```python
from build123d import *

# Parameters (mm, degrees)
EXTRUDE_1_DEPTH     = 5
EXTRUDE_2_DEPTH     = 15
CUT_EXTRUDE_1_DEPTH = 15


with BuildPart() as part:
    # 草圖1 → 填料-伸長1 (new body)
    with BuildSketch(Plane(origin=(0, 0, 0), x_dir=(1, 0, 0), z_dir=(0, 1, 0))):
        with BuildLine():
            ThreePointArc((-10, 5), (-15, 0), (-10, -5))
            Line((-10, -5), (0, -5))
            Line((0, -5), (0, -10))
            ThreePointArc((0, -10), (10, 0), (0, 10))
            Line((0, 10), (-5, 10))
            Line((-5, 10), (-5, 5))
            Line((-5, 5), (-10, 5))
        make_face()
    extrude(amount=EXTRUDE_1_DEPTH)

    # 草圖1<3> → 填料-伸長2 (add)
    with BuildSketch(Plane(origin=(0, 0, 0), x_dir=(1, 0, 0), z_dir=(0, 1, 0))):
        Polygon((-10, 15), (-10, 5), (-5, 5), (-5, 10), (-5, 15), align=None)
    extrude(amount=EXTRUDE_2_DEPTH)

    # 草圖2 → 除料-伸長1 (cut)
    with BuildSketch(Plane.ZY.offset(10)):
        Polygon((-15, 15), (-5, 5), (-5, 15), align=None)
    extrude(amount=-CUT_EXTRUDE_1_DEPTH, mode=Mode.SUBTRACT)


solid = part.part
```
Source: CAD feature listing. Evaluate the final solid. Frame: model axes, mm. A direction names the side the tool comes from. Coordinates: 2 decimals unless noted, no trailing zeros. Order: outer loops, then holes, each group sorted by start corner. A loop starts at its lowest first (then second) coordinate and runs counter-clockwise, first axis right, second up. Notation, with made-up numbers: M -39.75,58 L -19.75,58 A14 ccw -19.75,69 Z; hole C -28.5,32 d8. An arc over 180 degrees is marked long. Write each question's results on one line, items separated by ' | '. Start each with the question number.
1) Section query C-C (y = 7). Return the cut outline in (x, z).
2) Section query A-A (x = -9.5). Return the cut outline in (y, z).
3) Section query D-D (z = 0). Return the cut outline in (x, y), plus the area to 3 significant figures.
4) Line query: line 1 (Y direction, x = 4.5, z = 3); line 2 (X direction, y = 9.25, z = -13.5); line 3 (X direction, y = 3.5, z = -7.75). Output: solid intervals per line, ascending. Write a range as from..to.
5) Access query for faces 1 (the face through (-3, 0, -3)), 2 (the face through (0, 2, 7)), 3 (the face through (-2, 2, -10)), 4 (the face through (-3, 5, 0)), 5 (the face through (-10, 6, -11)). Directions: +Z, -Z, +X, -X, +Y, -Y. A direction counts if a zero-diameter tool reaches every point of the face in a straight line with its end or side. Return the directions, or none.
6) Section query B-B (z = -9). Return the cut outline in (x, y).
7) Contact query for flat-ended pins moving along their axis: pin 1 Ø1.5 at (x, y) = (-3, 3.5) entering from -Z; pin 2 Ø5 at (x, z) = (-5.5, -4) entering from -Y; pin 3 Ø5 at (y, z) = (10, -9) entering from +X; pin 4 Ø1.5 at (x, y) = (-7, 3) entering from +Z. Output: stop coordinate, or through.
Answers:
1) outline: M -10,-15 L -5,-15 L -5,-7 L -10,-7 Z
2) outline: M 0,-15 L 15,-15 L 5,-5 L 5,5 L 0,5 Z
3) outline: M -15,0 L 10,0 L 10,5 L -15,5 Z | area: 125 mm^2
4) line 1: y = 0..5 | line 2: x = -10..-5 | line 3: x = -10..6.32
5) face 1: +Z, -Z, +X, -X, -Y | face 2: +Z, -X, +Y, -Y | face 3: -Z, +X, +Y, -Y | face 4: +Z, +X, +Y | face 5: -Z, -X, +Y, -Y
6) outline: M -10,0 L 4.36,0 L 4.36,5 L -5,5 L -5,9 L -10,9 Z
7) pin 1: stops at z = -10 | pin 2: stops at y = 0 | pin 3: stops at x = -5 | pin 4: stops at z = 5
